```python
from build123d import *

# Parameters (mm, degrees)
F0_W      = 10
F0_H      = 14
F1_DEPTH  = 10
F2_R      = 2.1
F3_DEPTH  = 15
F4_R      = 0.9
F5_DEPTH  = 5
F6_R      = 2
F8_DEPTH  = 10
F9_R      = 2.5
F10_DEPTH = 5
F11_R     = 4.99999


# Not quite as in the source:
# - a fillet or chamfer is up to 0.001 mm smaller than in the source, because OpenCascade refuses the exact size


with BuildPart() as f1:
    # F0 (on Top) → F1 (new body)
    with BuildSketch(Plane.XY):
        Rectangle(F0_W, F0_H)
    extrude(amount=F1_DEPTH)

    # F2 (on face) → F3 (join)
    with BuildSketch(Plane(origin=(0, 7, 0), x_dir=(-1, 0, 0), z_dir=(0, 1, 0))):
        with Locations((0, 2.1)):
            Circle(F2_R)
    extrude(amount=F3_DEPTH)

    # F4 (on Top) → F5 (cut)
    with BuildSketch(Plane.XY):
        with Locations((0, 18)):
            Circle(F4_R)
    extrude(amount=F5_DEPTH, mode=Mode.SUBTRACT)

    # F6
    f6_edges = [f1.edges().sort_by_distance(p)[0] for p in [
        (2.1, 22, 2.1),
    ]]
    fillet(f6_edges, radius=F6_R)

    # F7 (on face) → F8 (cut)
    with BuildSketch(Plane(origin=(-5, 0, 0), x_dir=(0, -1, 0), z_dir=(-1, 0, 0))):
        Polygon((4, 10), (7, 0), (7, 10), align=None)
    extrude(amount=-F8_DEPTH, mode=Mode.SUBTRACT)

    # F9 (on face) → F10 (cut)
    with BuildSketch(Plane(origin=(0, -6.4220183486, 1.9266055046), x_dir=(1, 0, 0), z_dir=(0, -0.9578262852, 0.2873478856))):
        with Locations((0, 3.9318241179)):
            Circle(F9_R)
    extrude(amount=-F10_DEPTH, mode=Mode.SUBTRACT)

    # F11 (radius 5 in the source; OpenCascade refuses exactly that, so slightly less here)
    f11_edges = [f1.edges().sort_by_distance(p)[0] for p in [
        (-5, 1.5, 10),
        (5, 1.5, 10),
    ]]
    fillet(f11_edges, radius=F11_R)


solid = f1.part
```
Model file for the job. Use its own axes, mm. Coordinates: 2 decimals unless noted, no trailing zeros. Write each loop counter-clockwise with the first axis right and the second up, starting at its lowest first coordinate (ties: lowest second). Pieces come first, ordered by that corner, then holes. Notation, with made-up numbers: (24, 38.25) - (54, 38.25) arc R19 ccw to (54, 47.25) - close; hole circle Ø8 at (-18, 57.5). An arc over 180 degrees is marked (long way). Use a Markdown table: item, result. Add a question column.
Item 1: Drill centre lines: line 1 along X through (y, z) = (18, 2.1); line 2 along X through (y, z) = (18, 1.4); line 3 along Z through (x, y) = (-2, 0). Where is each one in solid material? Low to high.
Item 2: Band-saw the part on B-B, the plane x = -3.25. Write the cut outline in (y, z), and give its area (3 significant figures).
Item 3: Two-plate mould, pull along X, no slides. Class faces 1 (the face through (-0.035, -0.493, 4.289)), 2 (the face through (5, 0, 2)), 3 (the face through (-1.94, 13.41, 1.3)): pulls with the +X half, pulls with the -X half, needs draft (parallel to the pull), parting line crosses it, or undercut.
Item 4: Drop flat-ended pins along their axis: pin 1 (1.4 mm diameter, centred on x = 0, y = 18, fed in from +Z); pin 2 (6 mm diameter, centred on x = 1, z = 6, fed in from +Y); pin 3 (2 mm diameter, centred on x = 0, z = 2, fed in from -Y); pin 4 (2 mm diameter, centred on y = 1, z = 9, fed in from -X). Give the stop position or say it passes through.
Item 5: Band-saw the part on A-A, the plane y = 13.75. Write the cut outline in (x, z), and give its area (3 significant figures).
Item 6: Band-saw the part on C-C, the plane y = 18. Write the cut outline in (x, z).
A:
| question | item | result |
|---|---|---|
| 1 | line 1 | x = -2.1 to -0.9, 0.9 to 2.1 |
| 1 | line 2 | x = -1.98 to -0.9, 0.9 to 1.98 |
| 1 | line 3 | z = 0 to 9.58 |
| 2 | outline | (-7, 0) - (7, 0) - (7, 8.8) - (-4.36, 8.8) - close |
| 2 | area | 112 mm² |
| 3 | face 1 | undercut |
| 3 | face 2 | pulls with the +X half |
| 3 | face 3 | parting line crosses it |
| 4 | pin 1 | passes through |
| 4 | pin 2 | stops at y = 21.77 |
| 4 | pin 3 | stops at y = -6.7 |
| 4 | pin 4 | stops at x = -4 |
| 5 | outline | circle Ø4.2 at (0, 2.1) |
| 5 | area | 13.9 mm² |
| 6 | outline | (-0.9, 0.2) - (-0.9, 4) arc R2.1 ccw to start; (0.9, 0.2) arc R2.1 ccw to (0.9, 4) - close |
